Source: three-view drawing plus pictorial views. Frame: mm from the lowest corner of the part. Give positions to 0.01 mm unless a question says otherwise; leave off trailing zeros. Order: outer loops, then holes, each group sorted by start corner. A loop starts at its lowest first (then second) coordinate and runs counter-clockwise, first axis right, second up. Notation, with made-up numbers: (57.5, -11.75) - (82.5, -11.75) arc R9 ccw to (82.5, 1.25) - close; hole circle Ø10 at (5, 14.5). An arc over 180 degrees is marked (long way). Answer in a Markdown table with one row per item. Add a question column.
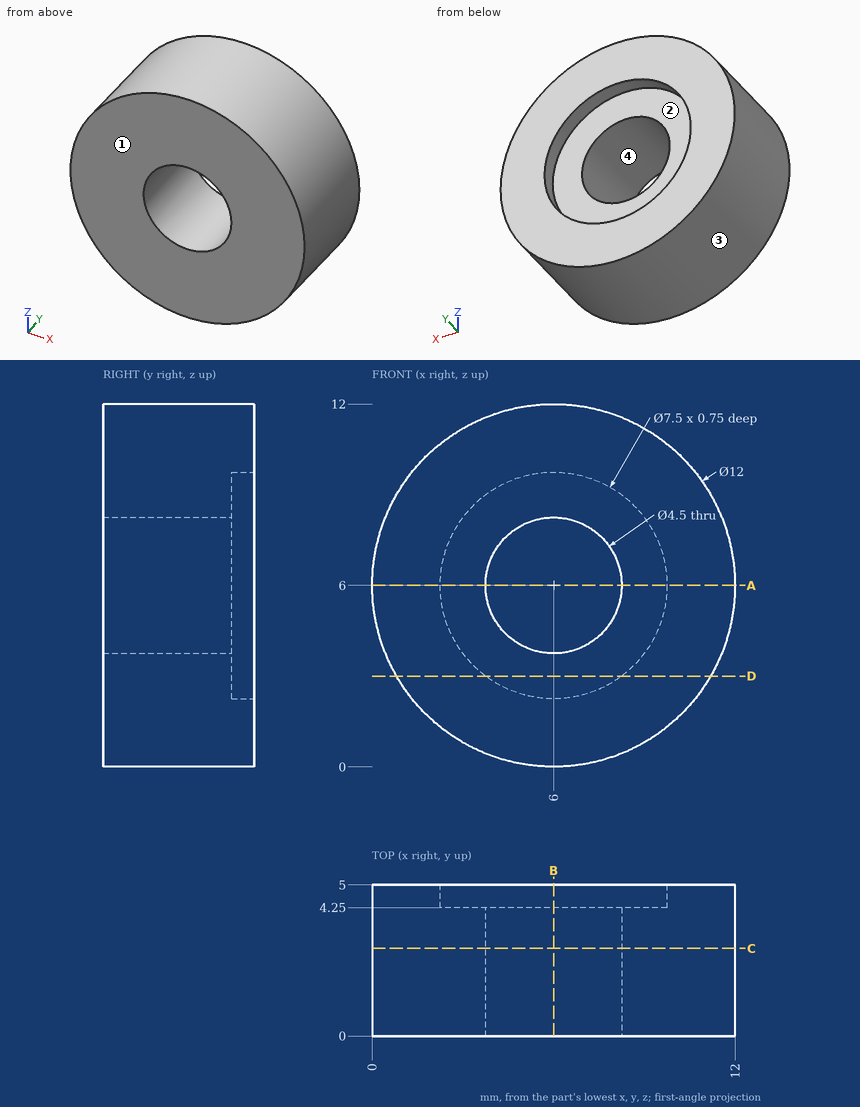
Q1. Line query: probe 1 along Z at (x, y) = (6, 4.75); probe 2 along Z at (x, y) = (6, 2.75). Output: solid intervals per line, ascending.
Q2. Section C-C, the plane y = 2.9. Return loops of the section in (x, z), then the cut area to 3 significant figures.
Q3. Section A-A, the plane z = 6. Return loops of the section in (x, y).
Q4. Section D-D, the plane z = 3. Return loops of the section in (x, y), then the cut area to 3 significant figures.
Q5. Section B-B, the plane x = 6. Return loops of the section in (y, z), then the cut area to 4 significant figures.
Q6. Contact query for a flat-ended pin moving along its axis: P1, Ø4, axis at x = 6, z = 6, coming from the +Y side. Output: stop coordinate, or through.
Q7. Pull-direction query (Z, two-part tool) for the marked faces 1, 2, 3 and 4; classes: +Z half, -Z half, draft (parallel to the pull), parting line (faces both ways), or undercut.
Computed:
| question | item | result |
|---|---|---|
| 1 | probe 1 | z = 0 to 2.25, 9.75 to 12 |
| 1 | probe 2 | z = 0 to 3.75, 8.25 to 12 |
| 2 | outline | circle Ø12 at (6, 6); hole circle Ø4.5 at (6, 6) |
| 2 | area | 97.2 mm^2 |
| 3 | outline | (0, 0) - (3.75, 0) - (3.75, 4.25) - (2.25, 4.25) - (2.25, 5) - (0, 5) - close; (8.25, 0) - (12, 0) - (12, 5) - (9.75, 5) - (9.75, 4.25) - (8.25, 4.25) - close |
| 4 | outline | (0.8, 0) - (11.2, 0) - (11.2, 5) - (8.25, 5) - (8.25, 4.25) - (3.75, 4.25) - (3.75, 5) - (0.8, 5) - close |
| 4 | area | 48.6 mm^2 |
| 5 | outline | (0, 0) - (5, 0) - (5, 2.25) - (4.25, 2.25) - (4.25, 3.75) - (0, 3.75) - close; (0, 8.25) - (4.25, 8.25) - (4.25, 9.75) - (5, 9.75) - (5, 12) - (0, 12) - close |
| 5 | area | 35.25 mm^2 |
| 6 | P1 | passes through |
| 7 | face 1 | draft |
| 7 | face 2 | undercut |
| 7 | face 3 | parting line |
| 7 | face 4 | undercut |
